from build123d import *

# Parameters (mm, degrees)
SKETCH012_R     = 12.2
PAD010_DEPTH    = 30.8
PAD011_DEPTH    = 8
SKETCH014_R     = 1
POCKET002_DEPTH = 5
SKETCH015_R     = 3.5
SKETCH015_R_2   = 2
PAD012_DEPTH    = 2.7


with BuildPart() as part:
    # Sketch012 → Pad010 (new body)
    with BuildSketch(Plane.XY):
        Circle(SKETCH012_R)
    extrude(amount=-PAD010_DEPTH)

    # Sketch013 → Pad011 (join)
    with BuildSketch(Plane.XY):
        with BuildLine():
            Line((-1.0535656252, 1.6999998451), (1.0535656252, 1.6999998451))
            ThreePointArc((0, -2), (1.9235383659, -0.5477226989), (1.0535656252, 1.6999998451))
            ThreePointArc((-1.0535656252, 1.6999998451), (-1.9235383659, -0.5477226989), (0, -2))
        make_face()
    extrude(amount=PAD011_DEPTH)

    # Sketch014 (on Face2 of Pad011) → Pocket002 (cut)
    with BuildSketch(Plane.XY):
        with Locations((-8.5, 0)):
            Circle(SKETCH014_R)
        with Locations((8.5, 0)):
            Circle(SKETCH014_R)
    extrude(amount=-POCKET002_DEPTH, mode=Mode.SUBTRACT)

    # Sketch015 (on Face2 of Pocket002) → Pad012 (join)
    with BuildSketch(Plane.XY):
        Circle(SKETCH015_R)
        Circle(SKETCH015_R_2, mode=Mode.SUBTRACT)
    extrude(amount=PAD012_DEPTH)


with BuildPart() as part_1:
    # Body003 placement: moved
    add(part.part.moved(Location((0, 0, -31))))


solid = part_1.part
The listing builds one solid part. Answer for the finished solid, in the listing's coordinates (mm). A direction names the side the tool comes from. Round coordinates to 2 decimals unless told otherwise and drop trailing zeros. Write each loop counter-clockwise with the first axis right and the second up, starting at its lowest first coordinate (ties: lowest second). Pieces come first, ordered by that corner, then holes. Notation, with made-up numbers: M -30.75,2.25 L -15.75,2.25 A28 ccw -15.75,27.25 Z; hole C 9,6.5 d7. An arc over 180 degrees is marked long. Write each question's results on one line, items separated by ' | '. Start each with the question number.
Item 1: Find section A-A on y = 0. Write down the section's boundary in (x, z), and give its area (3 significant figures).
Item 2: Given pin 1 Ø10 at (y, z) = (-5.5, -38.5) entering from +X; pin 2 Ø2 at (x, y) = (-6, -5) entering from +Z; pin 3 Ø4 at (y, z) = (8.5, -55) entering from -X, each flat-ended and moving along its own axis, determine where each tip first touches the part or whether it passes through.
Item 3: Which of the six approach directions +Z, -Z, +X, -X, +Y, -Y give full straight-line access (tool end or side, diameter ignored) to faces 1 (the cylindrical face through (3.233, -1.341, -29.669)), 2 (the flat face through (0, 0, -61.8))?
Item 4: Find section D-D on x = 8.5. Write down the section's boundary in (y, z), and give its area (3 significant figures).
Item 5: Find section B-B on x = 0. Write down the section's boundary in (y, z), and give its area (3 significant figures).
Item 6: Find section C-C on z = -39.5. Write down the section's boundary in (x, y), and give its area (3 significant figures).
Item 7: The mould has two halves that part along Y. Classify faces 3 (the flat face through (2, -2, -28.3)), 4 (the cylindrical face through (-12.19, 0.54, -46.18)), 5 (the cylindrical face through (-9.3, -0.6, -33.5)): +Y half, -Y half, draft (parallel to the pull), parting line (faces both ways), or undercut.
Item 8: Straight lines are drawn through the part: probe 1 along Z at (x, y) = (-7.75, 3.25); probe 2 along Y at (x, z) = (8.5, -33.4); probe 3 along Y at (x, z) = (0.25, -29). For each, find the intervals that lie inside material, in ascending order.
Answer block:
1) outline: M -12.2,-61.8 L 12.2,-61.8 L 12.2,-31 L 9.5,-31 L 9.5,-36 L 7.5,-36 L 7.5,-31 L 3.5,-31 L 3.5,-28.3 L 2,-28.3 L 2,-23 L -2,-23 L -2,-28.3 L -3.5,-28.3 L -3.5,-31 L -7.5,-31 L -7.5,-36 L -9.5,-36 L -9.5,-31 L -12.2,-31 Z | area: 772 mm²
2) pin 1: stops at x = 12.19 | pin 2: stops at z = -31 | pin 3: stops at x = -10.32
3) face 1: +Z | face 2: -Z, +X, -X, +Y, -Y
4) outline: M -8.75,-61.8 L 8.75,-61.8 L 8.75,-31 L 1,-31 L 1,-36 L -1,-36 L -1,-31 L -8.75,-31 Z | area: 529 mm²
5) outline: M -12.2,-61.8 L 12.2,-61.8 L 12.2,-31 L 3.5,-31 L 3.5,-28.3 L 2,-28.3 L 2,-31 L 1.7,-31 L 1.7,-23 L -2,-23 L -2,-28.3 L -3.5,-28.3 L -3.5,-31 L -12.2,-31 Z | area: 789 mm²
6) outline: C 0,0 d24.4 | area: 468 mm²
7) face 3: draft | face 4: parting line | face 5: undercut
8) probe 1: z = -61.8 to -31 | probe 2: y = -8.75 to -1, 1 to 8.75 | probe 3: y = -3.49 to 1.7, 1.98 to 3.49
